from build123d import *

# Parameters (mm, degrees)
F0_R      = 53.34
F0_R_2    = 22.225
F1_DEPTH  = 304.8
F4_R      = 53.34
F4_R_2    = 30.48
F5_DEPTH  = 101.6
F10_R     = 12.7
F10_R_2   = 8.89
F10_R_3   = 3.175
F11_DEPTH = 15.24
F12_DEPTH = 27.94
F13_DEPTH = 32.3429548439
F14_R     = 12.7
F14_R_2   = 8.89
F14_R_3   = 3.175
F15_DEPTH = 15.24
F16_DEPTH = 27.94
F17_DEPTH = 32.3429548439


with BuildPart() as f1:
    # F0 (on Front) → F1 (new body, symmetric)
    with BuildSketch(Plane.XZ):
        Circle(F0_R)
        Circle(F0_R_2, mode=Mode.SUBTRACT)
    extrude(amount=F1_DEPTH, both=True)

    # F4 (on offset) → F5 (cut)
    with BuildSketch(Plane(origin=(0, 304.8, 0), x_dir=(-1, 0, 0), z_dir=(0, 1, 0))):
        Circle(F4_R)
        Circle(F4_R_2, mode=Mode.SUBTRACT)
    extrude(amount=-F5_DEPTH, mode=Mode.SUBTRACT)

    # F6 (on Right) → F7 (revolve)
    with BuildSketch(Plane.YZ):
        Polygon((203.2, 53.34), (203.2, 30.48), (226.06, 30.48), align=None)
    revolve(axis=Axis((0, 101.6, 0), (0, 1, 0)))

    # F10 (on offset) → F11 (cut)
    with BuildSketch(Plane.XY.offset(53.34)):
        Circle(F10_R)
        Circle(F10_R_2, mode=Mode.SUBTRACT)
        Circle(F10_R_2)
        Circle(F10_R_3, mode=Mode.SUBTRACT)
        Circle(F10_R_3)
    extrude(amount=-F11_DEPTH, mode=Mode.SUBTRACT)

    # F10 (on offset) → F12 (cut)
    with BuildSketch(Plane.XY.offset(53.34)):
        Circle(F10_R_2)
        Circle(F10_R_3, mode=Mode.SUBTRACT)
        Circle(F10_R_3)
    extrude(amount=-F12_DEPTH, mode=Mode.SUBTRACT)

    # F10 (on offset) → F13 (cut, up to face)
    with BuildSketch(Plane.XY.offset(53.34)):
        Circle(F10_R_3)
    extrude(amount=-F13_DEPTH, mode=Mode.SUBTRACT)

    # F14 (on offset) → F15 (cut)
    with BuildSketch(Plane.XY.offset(-53.34)):
        Circle(F14_R)
        Circle(F14_R_2, mode=Mode.SUBTRACT)
        Circle(F14_R_2)
        Circle(F14_R_3, mode=Mode.SUBTRACT)
        Circle(F14_R_3)
    extrude(amount=F15_DEPTH, mode=Mode.SUBTRACT)

    # F14 (on offset) → F16 (cut)
    with BuildSketch(Plane.XY.offset(-53.34)):
        Circle(F14_R_2)
        Circle(F14_R_3, mode=Mode.SUBTRACT)
        Circle(F14_R_3)
    extrude(amount=F16_DEPTH, mode=Mode.SUBTRACT)

    # F14 (on offset) → F17 (cut, up to face)
    with BuildSketch(Plane.XY.offset(-53.34)):
        Circle(F14_R_3)
    extrude(amount=F17_DEPTH, mode=Mode.SUBTRACT)


solid = f1.part
Read the model definition and answer for the solid it produces. Units are mm, in the model's axes. A direction names the side the tool comes from. Give positions to 0.01 mm unless a question says otherwise; leave off trailing zeros. Write each loop counter-clockwise with the first axis right and the second up, starting at its lowest first coordinate (ties: lowest second). Pieces come first, ordered by that corner, then holes. Notation, with made-up numbers: (53, 68.5) -> (72, 68.5) arc R24 ccw to (72, 105.5) -> close; hole circle Ø11 at (85.25, 45). An arc over 180 degrees is marked (long way). Answer as a JSON object with one key per item and string values. Group by question number.
1) Each of these flat-tipped pins is pushed along its axis until it touches: P1, Ø23, axis at x = 0, y = 0, coming from the -Z side; P2, Ø12.5, axis at x = 0, y = -1.5, coming from the +Z side; P3, Ø2, axis at y = 139.5, z = -32, coming from the -X side. Where does it stop, or does it pass through?
2) A tool of negligible diameter and unlimited length cuts with its end or side. For faces 5 (the flat face through (23, -304.8, 1)), 6 (the cylindrical face through (12.114, 3.815, -45.827)), 7 (the cylindrical face through (-28.156, 265.981, -11.674)), 8 (the flat face through (2.1, 304.8, -22.4)), 9 (the cylindrical face through (-1.93, -8.68, 31.84)), from which of +Z, -Z, +X, -X, +Y, -Y can it reach the whole face along a straight path? Write none if from no direction.
3) Find section B-B (y = -175). Write down the section's boundary in (x, z) (3 decimals), and give its area (3 significant figures).
4) The mould has two halves that part along Z. Classify faces 1 (the flat face through (-9, -3, 38.1)), 2 (the cylindrical face through (21.199, 4.267, 6.676)), 3 (the flat face through (0, -4, -25.4)), 4 (the cylindrical face through (50.877, -54.356, 16.022)): +Z half, -Z half, draft (parallel to the pull), parting line (faces both ways), or undercut.
5) Consider L1, parallel to Y at x = 0, z = 24.4 (3 decimals); L2, parallel to Z at x = 2, y = 3; L3, parallel to Z at x = 0, y = -4 (3 decimals). Determine where each line is inside the solid, lowest interval first. Write a range as from..to.
6) Find section A-A (z = 0). Write down the section's boundary in (x, y) (3 decimals), and give its area (3 significant figures).
Values follow:
{
 "1": {"P1": "stops at z = -38.1", "P2": "stops at z = 25.4", "P3": "stops at x = -43.41"},
 "2": {"face 5": "+Z, -Z, +X, -X, -Y", "face 6": "-Z", "face 7": "+Y", "face 8": "+Z, -Z, +X, -X, +Y", "face 9": "+Z"},
 "3": {"outline": "circle Ø106.68 at (0, 0); hole circle Ø44.45 at (0, 0)", "area": "7,390 mm2"},
 "4": {"face 1": "+Z half", "face 2": "undercut", "face 3": "-Z half", "face 4": "parting line"},
 "5": {"L1": "y = -304.8..-3.175, 3.175..304.8", "L2": "z = -25.4..-22.13, 22.13..25.4", "L3": "z = -25.4..-22.225, 22.225..25.4"},
 "6": {"outline": "(-53.34, -304.8) -> (-22.225, -304.8) -> (-22.225, 304.8) -> (-30.48, 304.8) -> (-30.48, 226.06) -> (-53.34, 203.2) -> close; (22.225, -304.8) -> (53.34, -304.8) -> (53.34, 203.2) -> (30.48, 226.06) -> (30.48, 304.8) -> (22.225, 304.8) -> close", "area": "33,800 mm2"}
}
